Check sheet for the modelled part. Datum: model origin and axes. Units: mm. A direction names the side the tool comes from. Give positions to 0.01 mm unless a question says otherwise; leave off trailing zeros. Order: outer loops, then holes, each group sorted by start corner. A loop starts at its lowest first (then second) coordinate and runs counter-clockwise, first axis right, second up. Notation, with made-up numbers: (-39, -15) -> (2, -15) arc R16 ccw to (2, 12) -> close; hole circle Ø7 at (-27.75, 46). An arc over 180 degrees is marked (long way). Answer in a Markdown table with one row per item. Add a question column.
(1) Cross-section at D-D (x = -45.72). Record the cut outline in (y, z) (3 decimals).
(2) Release check for a two-part mould opening along Z. For faces 4 (the face through (-48.65, -5.03, -0.18)), 5 (the face through (1, 1, -12.7)), 6 (the face through (-1, 1, 12.7)), 7 (the face through (66.542, 10.208, -0.553)) record: released by +Z, released by -Z, zero draft, split by the parting line, or undercut.
(3) Cross-section at C-C (y = 76.2). Record the cut outline in (x, z).
(4) Cross-section at B-B (y = -3.81). Record the cut outline in (x, z) (3 decimals), then the cut area to 3 significant figures.
(5) Cross-section at A-A (x = 0). Record the cut outline in (y, z), then the cut area to 3 significant figures.
(6) Set-up check for faces 1 (the face through (-76.2, -1, 0)), 2 (the face through (66.542, -15.192, -0.553)), 3 (the face through (-66.542, 10.208, 0.553)): record each of +Z, -Z, +X, -X, +Y, -Y from which the full face is reachable in a straight line by a thin tool's end or side.
(7) Thickness scan on L1, parallel to Y at x = 45.72, z = -1.75 (3 decimals); L2, parallel to X at y = -38.1, z = 5.25; L3, parallel to Y at x = 0, z = -2.75. Record the ranges inside material, lowest first. Write a range as [from, to].
(8) Go/stop test with flat-tipped pins: pin 1 (4.5 mm diameter, centred on y = 12.7, z = 0, fed in from -X); pin 2 (3 mm diameter, centred on y = -62.5, z = -0.5, fed in from -X); pin 3 (4 mm diameter, centred on x = -29, z = -1.5, fed in from -Y). Record where each tip stops, or that it passes through.
```python
from build123d import *

# Parameters (mm, degrees)
SKETCH1_W                   = 177.8
SKETCH1_H                   = 177.8
EXTRUDE1_DEPTH              = 12.7
F_10_CLEARANCE_HOLE1_D      = 5.1054
CIRPATTERN1_COUNT           = 3
SKETCH5_W                   = 177.8
SKETCH5_H                   = 31.75
EXTRUDE2_DEPTH              = 1.5875
SKETCH8_R                   = 152.4
SKETCH8_R_2                 = 88.9
EXTRUDE3_DEPTH              = 13.7
SKETCH9_W                   = 254
SKETCH9_H                   = 254
SKETCH9_W_2                 = 152.4
SKETCH9_H_2                 = 177.8
EXTRUDE4_DEPTH              = 13.7
SKETCH10_W                  = 152.4
SKETCH10_H                  = 38.1
EXTRUDE5_DEPTH              = 12.7
EXTRUDE5_DEPTH_BACK         = 2.54
F_1_4_0_25_DIAMETER_HOLE1_D = 6.35
LPATTERN1_COUNT             = 2
LPATTERN1_PITCH             = 7.62
LPATTERN1_COUNT_DIR2        = 2
LPATTERN1_PITCH_DIR2        = 91.44
F_1_4_20_TAPPED_HOLE1_D     = 5.1054
F_1_4_20_TAPPED_HOLE1_DEPTH = 19.05
F_1_4_20_TAPPED_HOLE1_TIP   = 1.533817
F_1_4_20_TAPPED_HOLE2_D     = 5.1054
F_1_4_20_TAPPED_HOLE2_DEPTH = 19.05
F_1_4_20_TAPPED_HOLE2_TIP   = 1.533817
SKETCH17_R                  = 2.5527
EXTRUDE6_DEPTH              = 12.7


with BuildPart() as part:
    # Sketch1 → Extrude1 (new body)
    with BuildSketch(Plane.XY):
        Rectangle(SKETCH1_W, SKETCH1_H)
    extrude(amount=EXTRUDE1_DEPTH)

    # 10 Clearance Hole1 (through all)
    with Locations(Plane(origin=(0, 0, 0), x_dir=(-1, 0, 0), z_dir=(0, 0, -1))):
        with Locations((0, 76.2)):
            f_10_clearance_hole1 = Hole(F_10_CLEARANCE_HOLE1_D / 2)

    # CirPattern1: 10 Clearance Hole1 ×3 about axis
    cirpattern1_axis = Axis((0, 0, 0), (0, 0, 1))
    for i in range(1, CIRPATTERN1_COUNT):
        add(f_10_clearance_hole1.rotate(cirpattern1_axis, i * 360 / CIRPATTERN1_COUNT), mode=Mode.SUBTRACT)

    # Sketch5 → Extrude2 (cut)
    with BuildSketch(Plane.XY):
        Rectangle(SKETCH5_W, SKETCH5_H)
    extrude(amount=EXTRUDE2_DEPTH, mode=Mode.SUBTRACT)

    # Sketch8 → Extrude3 (cut, through all)
    with BuildSketch(Plane.XY.offset(12.7)):
        Circle(SKETCH8_R)
        Circle(SKETCH8_R_2, mode=Mode.SUBTRACT)
    extrude(amount=-EXTRUDE3_DEPTH, mode=Mode.SUBTRACT)

    # Sketch9 → Extrude4 (cut, through all)
    with BuildSketch(Plane.XY.offset(12.7)):
        Rectangle(SKETCH9_W, SKETCH9_H)
        Rectangle(SKETCH9_W_2, SKETCH9_H_2, mode=Mode.SUBTRACT)
    extrude(amount=-EXTRUDE4_DEPTH, mode=Mode.SUBTRACT)

    # Sketch10 → Extrude5 (add, two sides)
    with BuildSketch(Plane(origin=(0, 0, 0), x_dir=(-1, 0, 0), z_dir=(0, 0, -1))) as extrude5_sk:
        Rectangle(SKETCH10_W, SKETCH10_H)
    extrude(amount=EXTRUDE5_DEPTH)
    extrude(extrude5_sk.sketch, amount=-EXTRUDE5_DEPTH_BACK)

    # 1_4 _0.25_ Diameter Hole1 (through all)
    with Locations(Plane.XY.offset(12.7)):
        with Locations((-45.72, 3.81)):
            f_1_4_0_25_diameter_hole1 = Hole(F_1_4_0_25_DIAMETER_HOLE1_D / 2)

    # LPattern1: 1_4 _0.25_ Diameter Hole1 2 × 2
    with Locations(*[(j * LPATTERN1_PITCH_DIR2, -i * LPATTERN1_PITCH, 0) for i in range(LPATTERN1_COUNT) for j in range(LPATTERN1_COUNT_DIR2) if (i, j) != (0, 0)]):
        add(f_1_4_0_25_diameter_hole1, mode=Mode.SUBTRACT)

    # 1_4-20 Tapped Hole1
    with Locations(Plane.ZY.offset(76.2)):
        with Locations((0, 12.7), (0, -12.7)):
            Hole(F_1_4_20_TAPPED_HOLE1_D / 2, depth=F_1_4_20_TAPPED_HOLE1_DEPTH)
            with Locations((0, 0, -(F_1_4_20_TAPPED_HOLE1_DEPTH + F_1_4_20_TAPPED_HOLE1_TIP / 2))):  # 118° drill point
                Cone(0, F_1_4_20_TAPPED_HOLE1_D / 2, F_1_4_20_TAPPED_HOLE1_TIP, mode=Mode.SUBTRACT)

    # 1_4-20 Tapped Hole2
    with Locations(Plane(origin=(76.2, 0, 0), x_dir=(0, 0, -1), z_dir=(1, 0, 0))):
        with Locations((0, 12.7), (0, -12.7)):
            Hole(F_1_4_20_TAPPED_HOLE2_D / 2, depth=F_1_4_20_TAPPED_HOLE2_DEPTH)
            with Locations((0, 0, -(F_1_4_20_TAPPED_HOLE2_DEPTH + F_1_4_20_TAPPED_HOLE2_TIP / 2))):  # 118° drill point
                Cone(0, F_1_4_20_TAPPED_HOLE2_D / 2, F_1_4_20_TAPPED_HOLE2_TIP, mode=Mode.SUBTRACT)

    # Sketch17 → Extrude6 (add)
    with BuildSketch(Plane(origin=(0, 0, 0), x_dir=(-1, 0, 0), z_dir=(0, 0, -1))):
        with BuildLine():
            Line((76.2, -45.790501), (76.2, -19.05))
            Line((76.2, -19.05), (-76.2, -19.05))
            Line((-76.2, -19.05), (-76.2, -45.790501))
            ThreePointArc((-76.2, -45.790501), (0, -88.9), (76.2, -45.790501))
        make_face()
        with Locations((-65.991136, -38.1)):
            Circle(SKETCH17_R, mode=Mode.SUBTRACT)
        with Locations((65.991136, -38.1)):
            Circle(SKETCH17_R, mode=Mode.SUBTRACT)
        with BuildLine():
            Line((-76.2, 45.790501), (-76.2, 19.05))
            Line((-76.2, 19.05), (76.2, 19.05))
            Line((76.2, 19.05), (76.2, 45.790501))
            ThreePointArc((76.2, 45.790501), (0, 88.9), (-76.2, 45.790501))
        make_face()
        with Locations((0, 76.2)):
            Circle(SKETCH17_R, mode=Mode.SUBTRACT)
    extrude(amount=EXTRUDE6_DEPTH)


solid = part.part
```
Answer below:
| question | item | result |
|---|---|---|
| 1 | outline | (-76.242, -12.7) -> (-6.985, -12.7) -> (-6.985, 12.7) -> (-76.242, 12.7) -> close; (-0.635, -12.7) -> (0.635, -12.7) -> (0.635, 12.7) -> (-0.635, 12.7) -> close; (6.985, -12.7) -> (76.242, -12.7) -> (76.242, 12.7) -> (6.985, 12.7) -> close |
| 2 | face 4 | zero draft |
| 2 | face 5 | released by -Z |
| 2 | face 6 | released by +Z |
| 2 | face 7 | undercut |
| 3 | outline | (-45.79, -12.7) -> (-2.55, -12.7) -> (-2.55, 12.7) -> (-45.79, 12.7) -> close; (2.55, -12.7) -> (45.79, -12.7) -> (45.79, 12.7) -> (2.55, 12.7) -> close |
| 4 | outline | (-76.2, -12.7) -> (-48.895, -12.7) -> (-48.895, 12.7) -> (-76.2, 12.7) -> close; (-42.545, -12.7) -> (42.545, -12.7) -> (42.545, 12.7) -> (-42.545, 12.7) -> close; (48.895, -12.7) -> (76.2, -12.7) -> (76.2, 12.7) -> (48.895, 12.7) -> close |
| 4 | area | 3,550 mm² |
| 5 | outline | (-88.9, -12.7) -> (73.65, -12.7) -> (73.65, 12.7) -> (-88.9, 12.7) -> close; (78.75, -12.7) -> (88.9, -12.7) -> (88.9, 12.7) -> (78.75, 12.7) -> close |
| 5 | area | 4,390 mm² |
| 6 | face 1 | +Z, -Z, -X, +Y, -Y |
| 6 | face 2 | +X |
| 6 | face 3 | -X |
| 7 | L1 | y = [-76.242, -6.985], [-0.635, 0.635], [6.985, 76.242] |
| 7 | L2 | x = [-76.2, -68.54], [-63.44, 63.44], [68.54, 76.2] |
| 7 | L3 | y = [-88.9, 73.65], [78.75, 88.9] |
| 8 | pin 1 | stops at x = -56.97 |
| 8 | pin 2 | stops at x = -64.67 |
| 8 | pin 3 | stops at y = -84.7 |
